from build123d import *

# Parameters (mm, degrees)
F1_DEPTH = 10
F2_SIZE  = 1


with BuildPart() as f1:
    # F0 (on Top) → F1 (new body)
    with BuildSketch(Plane.XY):
        Polygon((5.730627, 32.5), (-5.730627, 32.5), (-16.500682, 28.58002), (-25.280512, 21.212868), (-31.011139, 11.287132), (-33.001365, 0), (-31.011139, -11.287132), (-25.280512, -21.212868), (-16.500682, -28.58002), (-5.730627, -32.5), (5.730627, -32.5), (16.500682, -28.58002), (25.280512, -21.212868), (31.011139, -11.287132), (33.001365, 0), (31.011139, 11.287132), (25.280512, 21.212868), (16.500682, 28.58002), align=None)
        Polygon((-13.962116, 24.183094), (-4.848992, 27.5), (4.848992, 27.5), (13.962116, 24.183094), (21.391203, 17.94935), (26.240195, 9.55065), (27.924232, 0), (26.240195, -9.55065), (21.391203, -17.94935), (13.962116, -24.183094), (4.848992, -27.5), (-4.848992, -27.5), (-13.962116, -24.183094), (-21.391203, -17.94935), (-26.240195, -9.55065), (-27.924232, 0), (-26.240195, 9.55065), (-21.391203, 17.94935), align=None, mode=Mode.SUBTRACT)
    extrude(amount=F1_DEPTH)

    # F2
    f2_edges = [f1.edges().sort_by_distance(p)[0] for p in [
        (-20.890597, 24.896444, 10),
        (-11.115655, 30.54001, 10),
        (0, 32.5, 10),
        (11.115655, 30.54001, 10),
        (20.890597, 24.896444, 10),
        (28.145826, 16.25, 10),
        (32.006252, 5.643566, 10),
        (32.006252, -5.643566, 10),
        (28.145826, -16.25, 10),
        (20.890597, -24.896444, 10),
        (11.115655, -30.54001, 10),
        (0, -32.5, 10),
        (-11.115655, -30.54001, 10),
        (-20.890597, -24.896444, 10),
        (-28.145826, -16.25, 10),
        (-32.006252, -5.643566, 10),
        (-32.006252, 5.643566, 10),
        (-28.145826, 16.25, 10),
        (-32.006252, 5.643566, 0),
        (-28.145826, 16.25, 0),
        (-20.890597, 24.896444, 0),
        (-11.115655, 30.54001, 0),
        (-32.006252, -5.643566, 0),
        (-28.145826, -16.25, 0),
        (-20.890597, -24.896444, 0),
        (-11.115655, -30.54001, 0),
        (0, -32.5, 0),
        (11.115655, -30.54001, 0),
        (20.890597, -24.896444, 0),
        (28.145826, -16.25, 0),
        (32.006252, -5.643566, 0),
        (32.006252, 5.643566, 0),
        (28.145826, 16.25, 0),
        (20.890597, 24.896444, 0),
        (11.115655, 30.54001, 0),
        (0, 32.5, 0),
    ]]
    chamfer(f2_edges, length=F2_SIZE)


solid = f1.part
Can you work these out from the model? Positions are in its coordinate system, mm. A direction names the side the tool comes from. Round coordinates to 2 decimals unless told otherwise and drop trailing zeros. Order: outer loops, then holes, each group sorted by start corner. A loop starts at its lowest first (then second) coordinate and runs counter-clockwise, first axis right, second up. Notation, with made-up numbers: M -11.5,56.5 L 46.5,56.5 A30 cw 46.5,87.5 Z; hole C -25.75,35 d9. An arc over 180 degrees is marked long. Use a Markdown table: item, result.
1) If we mould it in two halves opening along Y, with no side actions, what happens to faces 3 (the face through (20.626, 24.456, 9.507)), 4 (the face through (-17.625, -21.11, 4.93)), 5 (the face through (-20.952, -24.845, 4.944))? For each: +Y half, -Y half, draft (parallel to the pull), parting line (faces both ways), or undercut.
Geometry says:
| item | result |
|---|---|
| face 3 | +Y half |
| face 4 | undercut |
| face 5 | -Y half |
2) Imagine slicing it at A-A (x = 4). List the corners of the cut face in (y, z) for me, then the cut area to 3 significant figures.
Geometry says:
| item | result |
|---|---|
| outline | M -32.5,1 L -31.5,0 L -27.5,0 L -27.5,10 L -31.5,10 L -32.5,9 Z; M 27.5,0 L 31.5,0 L 32.5,1 L 32.5,9 L 31.5,10 L 27.5,10 Z |
| area | 98.0 mm² |
3) On a 3-axis mill with a long thin cutter (end or side, diameter ignored), from which of +Z, -Z, +X, -X, +Y, -Y can I reach the whole of each face in a straight line? I mean faces 1 (the face through (11.191, 30.513, 4.944)), 2 (the face through (9.47, -25.82, 4.93)). Say none if no direction works.
Geometry says:
| item | result |
|---|---|
| face 1 | +Z, -Z, +X, +Y |
| face 2 | +Z, -Z |
4) If I drill on line 1 along Y through (x, z) = (-2, 6.25); line 2 along X through (y, z) = (18.5, 3.25); line 3 along Y through (x, z) = (16, 6.75), over which ranges is the centre line in solid material (lowest first)?
Geometry says:
| item | result |
|---|---|
| line 1 | y = -32.5 to -27.5, 27.5 to 32.5 |
| line 2 | x = -26.85 to -20.73, 20.73 to 26.85 |
| line 3 | y = -28.76 to -22.47, 22.47 to 28.76 |
5) I'm going to push flat-ended pins straight in: P1, Ø3, axis at y = 19.5, z = 1.5, coming from the -X side; P2, Ø6, axis at y = 7, z = 8, coming from the -X side; P3, Ø6, axis at y = -3.5, z = 3.5, coming from the +X side. Where does each tip first touch, or does it pass through?
Geometry says:
| item | result |
|---|---|
| P1 | stops at x = -27.14 |
| P2 | stops at x = -32.3 |
| P3 | stops at x = 32.91 |
6) Imagine slicing it at B-B (y = 22.5). List the corners of the cut face in (x, z) for me.
Geometry says:
| item | result |
|---|---|
| outline | M -23.75,1 L -22.19,0 L -15.97,0 L -15.97,10 L -22.19,10 L -23.75,9 Z; M 15.97,0 L 22.19,0 L 23.75,1 L 23.75,9 L 22.19,10 L 15.97,10 Z |
